Model file for the job. Use its own axes, mm. Round coordinates to 2 decimals unless told otherwise and drop trailing zeros. Order: outer loops, then holes, each group sorted by start corner. A loop starts at its lowest first (then second) coordinate and runs counter-clockwise, first axis right, second up. Notation, with made-up numbers: (6, 9.25) -> (44, 9.25) arc R20 cw to (44, 35.25) -> close; hole circle Ø5 at (-1, -33.5). An arc over 180 degrees is marked (long way). Use CSV: the item, a comma, the result in double quotes.
Autodesk Fusion 360 part; units mm, degrees
sketch "Sketch1" plane through (0, 0, 0) normal (0, 0, 1) x (1, 0, 0)
  circle A0 centre (0, 0) radius 11.0625
  circle A1 centre (0, 0) radius 15
  line L0 (0, 0) -> (130, 0)
  circle A2 centre (130, 0) radius 11.0625
  circle A3 centre (130, 0) radius 15
  line L1 (0, 0) -> (65, 0)
  spline S0 degree 5 poles (7.4528, 13.0175) (7.8836, 12.9141) (8.7411, 12.7102) (10.015, 12.4132) (11.688, 12.0352) (13.7317, 11.594) (15.7226, 11.1861) (17.6579, 10.8135) (19.5392, 10.4779) (21.3761, 10.1803) (23.1841, 9.9205) (24.9799, 9.6971) (26.7778, 9.5065) (28.5855, 9.3432) (30.3994, 9.1985) (32.2092, 9.0627) (34.0044, 8.9273) (35.7794, 8.7866) (37.5401, 8.6406) (39.3083, 8.496) (41.1126, 8.3625) (42.9802, 8.2492) (44.9302, 8.1618) (46.9629, 8.0975) (49.0581, 8.0448) (51.1857, 7.988) (52.8875, 7.9263) (54.152, 7.865) (54.9881, 7.8168) (55.4044, 7.7909) knots 0 0 0 0 0 0 0.04 0.08 0.12 0.16 0.2 0.24 0.28 0.32 0.36 0.4 0.44 0.48 0.52 0.56 0.6 0.64 0.68 0.72 0.76 0.8 0.84 0.88 0.92 0.96 1 1 1 1 1 1
  line L2 (65, 0) -> (65, 43.1808)
  spline S1 degree 5 poles (55.4044, 7.7909) (55.7874, 7.7593) (56.5538, 7.7035) (57.7049, 7.642) (59.2419, 7.5975) (61.1644, 7.58) (62.701, 7.5793) (63.8515, 7.5799) (64.6173, 7.5801) (65, 7.5801) knots 0 0 0 0 0 0 0.2 0.4 0.6 0.8 1 1 1 1 1 1
  spline S2 degree 5 poles (122.5472, 13.0175) (122.1164, 12.9141) (121.2589, 12.7102) (119.985, 12.4132) (118.312, 12.0352) (116.2683, 11.594) (114.2774, 11.1861) (112.3421, 10.8135) (110.4608, 10.4779) (108.6239, 10.1803) (106.8159, 9.9205) (105.0201, 9.6971) (103.2222, 9.5065) (101.4145, 9.3432) (99.6006, 9.1985) (97.7908, 9.0627) (95.9956, 8.9273) (94.2206, 8.7866) (92.4599, 8.6406) (90.6917, 8.496) (88.8874, 8.3625) (87.0198, 8.2492) (85.0698, 8.1618) (83.0371, 8.0975) (80.9419, 8.0448) (78.8143, 7.988) (77.1125, 7.9263) (75.848, 7.865) (75.0119, 7.8168) (74.5956, 7.7909) knots 0 0 0 0 0 0 0.04 0.08 0.12 0.16 0.2 0.24 0.28 0.32 0.36 0.4 0.44 0.48 0.52 0.56 0.6 0.64 0.68 0.72 0.76 0.8 0.84 0.88 0.92 0.96 1 1 1 1 1 1
  line L3 (2.3089, 14.2524) -> (12.5967, 11.7826)
  line L4 (50.4549, 8.0994) -> (60.354, 7.4823)
  line L5 (127.6911, 14.2524) -> (117.4033, 11.7826)
  line L6 (79.5451, 8.0994) -> (69.646, 7.4823)
  spline S3 degree 5 poles (74.5956, 7.7909) (74.2126, 7.7593) (73.4462, 7.7035) (72.2951, 7.642) (70.7581, 7.5975) (68.8356, 7.58) (67.299, 7.5793) (66.1485, 7.5799) (65.3827, 7.5801) (65, 7.5801) knots 0 0 0 0 0 0 0.2 0.4 0.6 0.8 1 1 1 1 1 1
  line L7 (54.4257, 7.8715) -> (56.3832, 7.7102)
  line L8 (64.0213, 7.5801) -> (65.9787, 7.5801)
  line L9 (75.5743, 7.8715) -> (73.6168, 7.7102)
  line L10 (65.9787, 7.5801) -> (64.0213, 7.5801)
  spline S4 degree 5 poles (122.5472, -13.0175) (122.1164, -12.9141) (121.2589, -12.7102) (119.985, -12.4132) (118.312, -12.0352) (116.2683, -11.594) (114.2774, -11.1861) (112.3421, -10.8135) (110.4608, -10.4779) (108.6239, -10.1803) (106.8159, -9.9205) (105.0201, -9.6971) (103.2222, -9.5065) (101.4145, -9.3432) (99.6006, -9.1985) (97.7908, -9.0627) (95.9956, -8.9273) (94.2206, -8.7866) (92.4599, -8.6406) (90.6917, -8.496) (88.8874, -8.3625) (87.0198, -8.2492) (85.0698, -8.1618) (83.0371, -8.0975) (80.9419, -8.0448) (78.8143, -7.988) (77.1125, -7.9263) (75.848, -7.865) (75.0119, -7.8168) (74.5956, -7.7909) knots 0 0 0 0 0 0 0.04 0.08 0.12 0.16 0.2 0.24 0.28 0.32 0.36 0.4 0.44 0.48 0.52 0.56 0.6 0.64 0.68 0.72 0.76 0.8 0.84 0.88 0.92 0.96 1 1 1 1 1 1
  line L11 (127.6911, -14.2524) -> (117.4033, -11.7826)
  line L12 (79.5451, -8.0994) -> (69.646, -7.4823)
  spline S5 degree 5 poles (74.5956, -7.7909) (74.2126, -7.7593) (73.4462, -7.7035) (72.2951, -7.642) (70.7581, -7.5975) (68.8356, -7.58) (67.299, -7.5793) (66.1485, -7.5799) (65.3827, -7.5801) (65, -7.5801) knots 0 0 0 0 0 0 0.2 0.4 0.6 0.8 1 1 1 1 1 1
  line L13 (75.5743, -7.8715) -> (73.6168, -7.7102)
  line L14 (65.9787, -7.5801) -> (64.0213, -7.5801)
  spline S6 degree 5 poles (55.4044, -7.7909) (55.7874, -7.7593) (56.5538, -7.7035) (57.7049, -7.642) (59.2419, -7.5975) (61.1644, -7.58) (62.701, -7.5793) (63.8515, -7.5799) (64.6173, -7.5801) (65, -7.5801) knots 0 0 0 0 0 0 0.2 0.4 0.6 0.8 1 1 1 1 1 1
  line L15 (54.4257, -7.8715) -> (56.3832, -7.7102)
  line L16 (64.0213, -7.5801) -> (65.9787, -7.5801)
  spline S7 degree 5 poles (7.4528, -13.0175) (7.8836, -12.9141) (8.7411, -12.7102) (10.015, -12.4132) (11.688, -12.0352) (13.7317, -11.594) (15.7226, -11.1861) (17.6579, -10.8135) (19.5392, -10.4779) (21.3761, -10.1803) (23.1841, -9.9205) (24.9799, -9.6971) (26.7778, -9.5065) (28.5855, -9.3432) (30.3994, -9.1985) (32.2092, -9.0627) (34.0044, -8.9273) (35.7794, -8.7866) (37.5401, -8.6406) (39.3083, -8.496) (41.1126, -8.3625) (42.9802, -8.2492) (44.9302, -8.1618) (46.9629, -8.0975) (49.0581, -8.0448) (51.1857, -7.988) (52.8875, -7.9263) (54.152, -7.865) (54.9881, -7.8168) (55.4044, -7.7909) knots 0 0 0 0 0 0 0.04 0.08 0.12 0.16 0.2 0.24 0.28 0.32 0.36 0.4 0.44 0.48 0.52 0.56 0.6 0.64 0.68 0.72 0.76 0.8 0.84 0.88 0.92 0.96 1 1 1 1 1 1
  line L17 (2.3089, -14.2524) -> (12.5967, -11.7826)
  line L18 (50.4549, -8.0994) -> (60.354, -7.4823)
  ellipse E0 centre (65, 0) end of major axis (25, 0) minor radius 4
  line L19 (105, 0) -> (25, 0) construction
  line L20 (65, 4) -> (65, -4) construction
  point P0 (18.3178, 10.6996)
  point P1 (27.044, 9.4876)
  point P2 (35.5289, 8.8053)
  point P3 (44.207, 8.1979)
  point P4 (111.6822, 10.6996)
  point P5 (102.956, 9.4876)
  point P6 (94.4711, 8.8053)
  point P7 (85.793, 8.1979)
  point P8 (111.6822, -10.6996)
  point P9 (102.956, -9.4876)
  point P10 (94.4711, -8.8053)
  point P11 (85.793, -8.1979)
  point P12 (18.3178, -10.6996)
  point P13 (27.044, -9.4876)
  point P14 (35.5289, -8.8053)
  point P15 (44.207, -8.1979)
  dimension "d1" = 22.125
  dimension "d2" = 30
  dimension "d3" = 130
  dimension "d4" = 22.125
  dimension "d5" = 30
  dimension "d6" = 65
extrude "Extrude1" add sketch "Sketch1" along normal blind 7.142 contours A1 | A1 L0 L1 S0 L2 S1 L8 L10 E0 | A1 L0 A3 L1 S4 S5 L14 S6 L16 S7 E0 | L0 A3 L2 S2 S3 L8 L10 E0 | A3
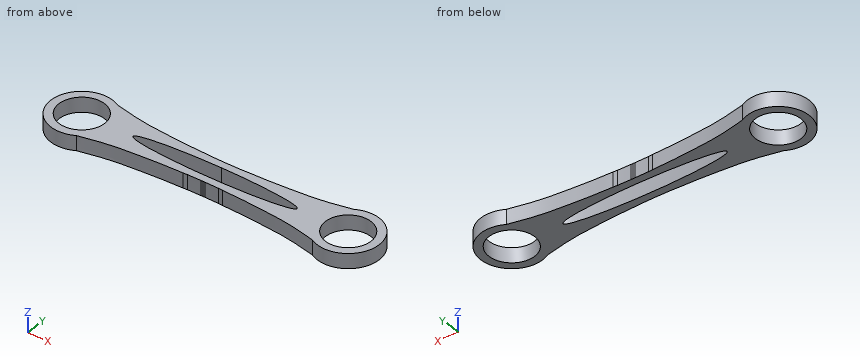
Q1. Pin check, flat tips, straight feed: pin 1 (0.5 mm diameter, centred on x = 64.5, z = 4.5, fed in from -Y); pin 2 (2 mm diameter, centred on y = -11.5, z = 3.5, fed in from +X). Stop position of each tip, or through.
From the geometry:
pin 1,"stops at y = -7.58"
pin 2,"stops at x = 140.71"
Q2. Cut at C-C (x = 127.5). Give the cut face in (y, z).
From the geometry:
outline,"(-14.79, 0) -> (-10.78, 0) -> (-10.78, 7.14) -> (-14.79, 7.14) -> close; (10.78, 0) -> (14.79, 0) -> (14.79, 7.14) -> (10.78, 7.14) -> close"
Q3. Cut at A-A (x = 0). Give the cut face in (y, z).
From the geometry:
outline,"(-15, 0) -> (-11.06, 0) -> (-11.06, 7.14) -> (-15, 7.14) -> close; (11.06, 0) -> (15, 0) -> (15, 7.14) -> (11.06, 7.14) -> close"
Q4. Cut at B-B (y = -6). Give the cut face in (x, z).
From the geometry:
outline,"(-13.75, 0) -> (-9.29, 0) -> (-9.29, 7.14) -> (-13.75, 7.14) -> close; (9.29, 0) -> (120.71, 0) -> (120.71, 7.14) -> (9.29, 7.14) -> close; (139.29, 0) -> (143.75, 0) -> (143.75, 7.14) -> (139.29, 7.14) -> close"
Q5. Cut at D-D (z = 1.75). State how many separate pieces and enclosed holes the cut face has, plus the area to 3 significant figures.
From the geometry:
separate pieces,"1"
enclosed holes,"3"
area,"1,980 mm²"
Q6. Probe line 1 along Y through (x, z) = (0, 3); line 2 along Y through (x, z) = (69, 1.75); line 3 along X through (y, z) = (-5.5, 6.25). List the from-to ranges inside material, lowest first.
From the geometry:
line 1,"y = -15 to -11.06, 11.06 to 15"
line 2,"y = -7.59 to -3.98, 3.98 to 7.59"
line 3,"x = -13.96 to -9.6, 9.6 to 120.4, 139.6 to 143.96"
